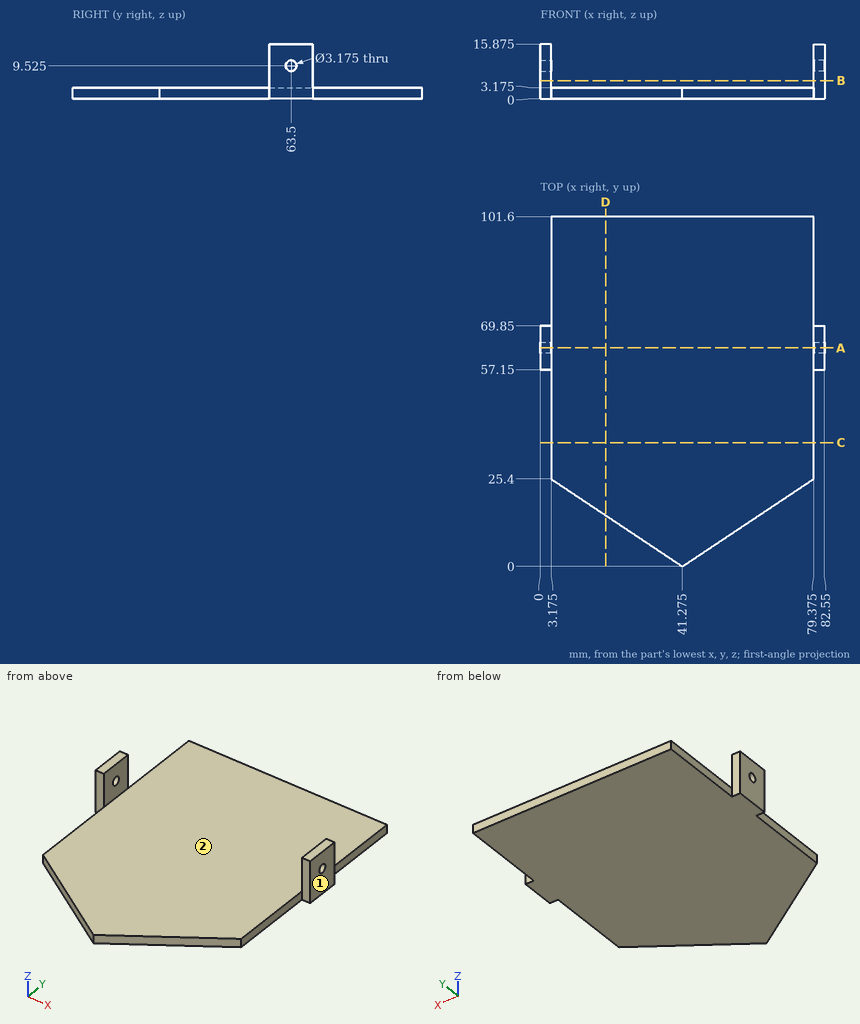
Part print with two shaded views. Sizes in mm from the minimum x, y, z corner. A direction names the side the tool comes from. Round coordinates to 2 decimals unless told otherwise and drop trailing zeros. Order: outer loops, then holes, each group sorted by start corner. A loop starts at its lowest first (then second) coordinate and runs counter-clockwise, first axis right, second up. Notation, with made-up numbers: (-14, 75) - (-1, 75) arc R7 cw to (-1, 79) - close; hole circle Ø4 at (-40, -22). An arc over 180 degrees is marked (long way). Return JSON: item names as keys, results as strings.
(1) Tool access for the marked faces 1 and 2: list every direction of +Z, -Z, +X, -X, +Y, -Y with a clear straight run to the whole face (end or side of a thin tool).
Answer key:
{"face 1": "+Z, -Z, +X, +Y, -Y", "face 2": "+Z, +Y, -Y"}
(2) Cut at D-D (x = 19). Give the cut face in (y, z) (3 decimals), then the cut area to 3 significant figures.
Answer key:
{"outline": "(14.85, 0) - (101.6, 0) - (101.6, 3.175) - (14.85, 3.175) - close", "area": "275 mm^2"}
(3) Pin check, flat tips, straight feed: pin 1 Ø3.5 at (y, z) = (90, 2) entering from +X (3 decimals); pin 2 Ø2.5 at (x, z) = (2, 11.5) entering from -Y; pin 3 Ø1 at (y, z) = (88.5, 1.5) entering from -X (3 decimals); pin 4 Ø6 at (y, z) = (27, 7.5) entering from -X. Stop position of each tip, or through.
Answer key:
{"pin 1": "stops at x = 79.375", "pin 2": "stops at y = 57.15", "pin 3": "stops at x = 3.175", "pin 4": "passes through"}
(4) Wall check: probe 1 along X at (y, z) = (59.5, 9.75) (3 decimals); probe 2 along Z at (x, y) = (1.9, 63.5) (1 decimal); probe 3 along Z at (x, y) = (40.5, 54) (3 decimals). Give the ranges that are in metal, low to high. Write a range as from..to.
Answer key:
{"probe 1": "x = 0..3.175, 79.375..82.55", "probe 2": "z = 0..7.9, 11.1..15.9", "probe 3": "z = 0..3.175"}
(5) Cut at C-C (y = 36). Give the cut face in (x, z) (3 decimals), then the cut area to 3 significant figures.
Answer key:
{"outline": "(3.175, 0) - (79.375, 0) - (79.375, 3.175) - (3.175, 3.175) - close", "area": "242 mm^2"}
(6) Cut at B-B (z = 5.25). Give the cut face in (x, y) (3 decimals), then the cut area to 3 significant figures.
Answer key:
{"outline": "(0, 57.15) - (3.175, 57.15) - (3.175, 69.85) - (0, 69.85) - close; (79.375, 57.15) - (82.55, 57.15) - (82.55, 69.85) - (79.375, 69.85) - close", "area": "80.6 mm^2"}
(7) Cut at A-A (y = 63.5). State how many separate pieces and enclosed holes the cut face has, then the cut area to 3 significant figures.
Answer key:
{"separate pieces": "3", "enclosed holes": "0", "area": "323 mm^2"}
